Autodesk Inventor part; units mm, degrees
ref_plane "YZ Plane" through (0, 0, 0) normal (1, 0, 0) x (0, 1, 0)
ref_plane "XZ Plane" through (0, 0, 0) normal (0, 1, 0) x (-1, 0, 0)
ref_plane "XY Plane" through (0, 0, 0) normal (0, 0, 1) x (1, 0, 0)
sketch "Sketch1" plane through (0, 0, 0) normal (0, 0, 1) x (1, 0, 0)
  line L0 (10, 4.75) -> (-10, 4.75)
  line L1 (-10, 4.75) -> (-10, -4.75)
  line L2 (-10, -4.75) -> (10, -4.75)
  line L3 (10, -4.75) -> (10, 4.75)
  line L4 (0.25, -4.75) -> (0.25, -5.45)
  line L5 (0.25, -5.45) -> (10, -5.45)
  line L6 (10, -5.45) -> (10, -4.75)
  line L7 (-10, -4.75) -> (10, 4.75) construction
  line L8 (10, -4.75) -> (-10, 4.75) construction
  circle A0 centre (-4.75, 2.25) radius 1.27
  circle A1 centre (4.75, 2.25) radius 1.27
  line L9 (0, 0) -> (0, 4.75) construction
  dimension "d0" = 20
  dimension "d2" = 10.2
  dimension "d3" = 9.5
  dimension "d4" = 9.75
  dimension "d5" = 9.5
  dimension "d6" = 2.54
  dimension "d7" = 2.5
extrude "Extrusion1" add sketch "Sketch1" along normal mid plane 6
sketch "Sketch2" plane through (0.25, -5.45, -3) normal (0, -1, 0) x (1, 0, 0)
  line L0 (6.75, 0.9) -> (6.25, 0.9)
  line L1 (6.25, 0.9) -> (6.25, 5.1)
  line L2 (6.25, 5.1) -> (6.75, 5.1)
  line L3 (6.75, 5.1) -> (6.75, 0.9)
  line L4 (-14.25, 3) -> (13.75, 3)
  line L5 (9.75, 0) -> (9.75, 6)
  point P0 (-0.25, 3)
  dimension "d10" = 4.2
  dimension "d11" = 0.5
  dimension "d12" = 3
extrude "Extrusion2" add sketch "Sketch2" along normal blind 1
sketch "Sketch3" plane through (6.5, -5.45, 2.1) normal (0, 0, 1) x (1, 0, 0)
  line L0 (0, -1) -> (-20.256, -4.1472)
  line L1 (-20.256, -4.1472) -> (-20.1793, -4.6413)
  line L2 (-20.1793, -4.6413) -> (0.0768, -1.4941)
  arc A0 (0.0768, -1.4941) -> (0.5, -1) centre (0, -1) ccw
  line L3 (0.5, -1) -> (0, -1)
  point P0 (-6.5, 5.45)
  dimension "d15" = 0.5
extrude "Extrusion3" add sketch "Sketch3" against normal blind 4.2
properties part number "Limit Switch"
Can you work these out from the model? Positions are in its coordinate system, mm. A direction names the side the tool comes from. Coordinates: 2 decimals unless noted, no trailing zeros. Loops run counter-clockwise (first coordinate to the right, second up) from the corner with the lowest first, then second, coordinate; pieces in that order, holes last.
1) Imagine slicing it at D-D on z = -0.2. List the corners of the cut face in (x, y) for me, plus the area to 3 significant figures.
2) Imagine slicing it at A-A on z = 2.35. List the corners of the cut face in (x, y) for me, plus the area to 3 significant figures.
3) For pin 1 (1 mm diameter, centred on x = -10, z = 0, fed in from -Y); pin 2 (1.8 mm diameter, centred on x = -3, z = 0.5, fed in from -Y); pin 3 (1.5 mm diameter, centred on x = -7, z = 0, fed in from -Y); pin 4 (2 mm diameter, centred on x = -4.75, y = 2.25, fed in from +Z), each with a flat end and sliding along its axis, tell me the tip position at first contact or that it passes through.
4) Thinking about a two-plate mould opening in X: for faces 1 (the flat face through (-5, -4.75, 0)), 2 (the flat face through (-3.486, -8.002, 0.029)), 3 (the cylindrical face through (5.96, 1.87, -0.04)), which applies, pulls with the +X half, pulls with the -X half, needs draft (parallel to the pull), parting line crosses it, or undercut?
5) Imagine slicing it at C-C on x = 5.25. List the corners of the cut face in (y, z) for me, plus the area to 3 significant figures.
6) Which directions (+Z, -Z, +X, -X, +Y, -Y) give clear straight access to the entire face, cutting with the end or side of a thin tool? Please do faces 4 (the flat face through (7, -6, 0)), 5 (the flat face through (-10, 0, 0)), 6 (the flat face through (-2.7, -8.1, 2.1)).
7) I need wall thicknesses on probe 1 along Y at (x, z) = (-4.75, 1.55); probe 2 along X at (y, z) = (1.75, 1.95); probe 3 along Y at (x, z) = (4.75, -0.2). Which ranges of each line are inside material? Lowest first, please.
8) Imagine slicing it at B-B on y = 2.25. List the corners of the cut face in (x, z) for me.
Completed:
1. outline: (-13.76, -9.6) - (-13.68, -10.09) - (6.58, -6.94) arc R0.5 ccw to (7, -6.45) - (7, -5.45) - (10, -5.45) - (10, 4.75) - (-10, 4.75) - (-10, -4.75) - (0.25, -4.75) - (0.25, -5.45) - (6.5, -5.45) - (6.5, -6.45) - close; hole circle Ø2.54 at (-4.75, 2.25); hole circle Ø2.54 at (4.75, 2.25)
1. area: 198 mm2
2. outline: (-10, -4.75) - (0.25, -4.75) - (0.25, -5.45) - (10, -5.45) - (10, 4.75) - (-10, 4.75) - close; hole circle Ø2.54 at (-4.75, 2.25); hole circle Ø2.54 at (4.75, 2.25)
2. area: 187 mm2
3. pin 1: stops at y = -9.6
3. pin 2: stops at y = -8.57
3. pin 3: stops at y = -9.17
3. pin 4: passes through
4. face 1: needs draft
4. face 2: pulls with the -X half
4. face 3: undercut
5. outline: (-7.15, -2.1) - (-6.64, -2.1) - (-6.64, 2.1) - (-7.15, 2.1) - close; (-5.45, -3) - (1.08, -3) - (1.08, 3) - (-5.45, 3) - close; (3.42, -3) - (4.75, -3) - (4.75, 3) - (3.42, 3) - close
5. area: 49.3 mm2
6. face 4: +Z, -Z, +X, -Y
6. face 5: +Z, -Z, -X, +Y
6. face 6: +Z, +X, -X, -Y
7. probe 1: y = -8.7 to -8.2, -4.75 to 0.98, 3.52 to 4.75
7. probe 2: x = -10 to -5.92, -3.58 to 3.58, 5.92 to 10
7. probe 3: y = -7.23 to -6.72, -5.45 to 0.98, 3.52 to 4.75
8. outline: (-10, -3) - (-6.02, -3) - (-6.02, 3) - (-10, 3) - close; (-3.48, -3) - (3.48, -3) - (3.48, 3) - (-3.48, 3) - close; (6.02, -3) - (10, -3) - (10, 3) - (6.02, 3) - close
